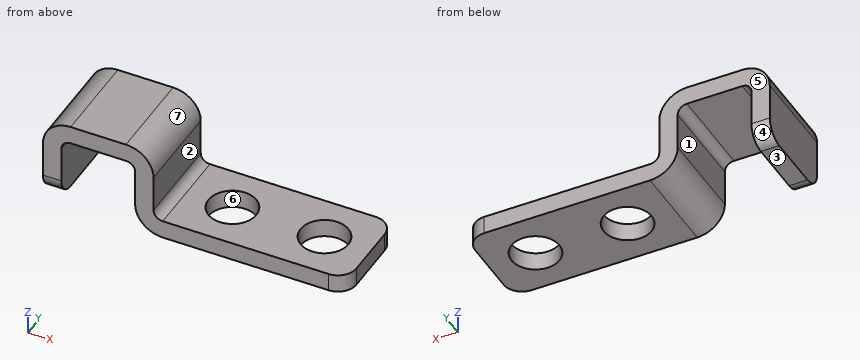
from build123d import *

# Parameters (mm, degrees)
F1_W = 10
F1_H = 2
F3_R = 2
F4_R = 2
F6_D = 5.2


with BuildPart() as f2:
    # F2: sweep along a path in F0
    with BuildLine(Plane.XZ) as f2_path:
        Line((0, 0), (-20, 0))
        ThreePointArc((-20, 0), (-21.4142135624, 0.5857864376), (-22, 2))
        Line((-22, 2), (-22, 6))
        ThreePointArc((-22, 6), (-22.5857864376, 7.4142135624), (-24, 8))
        Line((-24, 8), (-30, 8))
        ThreePointArc((-30, 8), (-31.4142135624, 7.4142135624), (-32, 6))
        Line((-32, 6), (-32, 0))
    # F1 (on Right) → F2 (sweep)
    with BuildSketch(Plane.YZ):
        with Locations((5, 0)):
            Rectangle(F1_W, F1_H)
    sweep(path=f2_path.line)

    # F3
    f3_edges = [f2.edges().sort_by_distance(p)[0] for p in [
        (-32, 0, 0),
        (-32, 10, 0),
    ]]
    fillet(f3_edges, radius=F3_R)

    # F4
    f4_edges = [f2.edges().sort_by_distance(p)[0] for p in [
        (0, 0, 0),
        (0, 10, 0),
    ]]
    fillet(f4_edges, radius=F4_R)

    # F6 (through all)
    with Locations(Plane.XY.offset(1)):
        with Locations((-15, 5), (-5, 5)):
            Hole(F6_D / 2)


solid = f2.part
The listing builds one solid part. Answer for the finished solid, in the listing's coordinates (mm). Face numbers are marked on the shaded views. A direction names the side the tool comes from. Coordinates: 2 decimals unless noted, no trailing zeros. Loops run counter-clockwise (first coordinate to the right, second up) from the corner with the lowest first, then second, coordinate; pieces in that order, holes last.
1) Determine the mould class of the marked faces 5, 6 and 7 for opening direction Y: pulls with the +Y half, pulls with the -Y half, needs draft (parallel to the pull), parting line crosses it, or undercut.
2) Find section A-A on x = -4. Write down the section's boundary in (y, z).
3) Find section B-B on y = 2.75. Write down the section's boundary in (x, z).
4) Flat-ended cylindrical pins translate along their axes: pin 1 Ø1.2 at (y, z) = (4.5, 3.5) entering from +X; pin 2 Ø2 at (x, y) = (-32.5, 6.5) entering from -Z; pin 3 Ø4 at (x, z) = (-26, 2.5) entering from -Y; pin 4 Ø3 at (x, y) = (-12, 5.5) entering from +Z. Find the tip coordinate at first contact, or state that the pin passes through.
5) Find section D-D on y = 6. Write down the section's boundary in (x, z).
6) Find section C-C on z = 6.5. Write down the section's boundary in (x, y).
7) Find the intervals of material crossed by L1, parallel to X at y = 0.5, z = 4; L2, parallel to Y at x = -5, z = 0.25; L3, parallel to Z at x = -29, y = 7, in increasing order.
8) A tool of negligible diameter and unlimited length cuts with its end or side. For the marked faces 1, 2, 3 and 4, from which of +Z, -Z, +X, -X, +Y, -Y can it reach the whole face along a straight path? Write none if from no direction.
Values:
1. face 5: pulls with the +Y half
1. face 6: undercut
1. face 7: needs draft
2. outline: (0, -1) - (2.6, -1) - (2.6, 1) - (0, 1) - close; (7.4, -1) - (10, -1) - (10, 1) - (7.4, 1) - close
3. outline: (-33, 0) - (-31, 0) - (-31, 6) arc R1 cw to (-30, 7) - (-24, 7) arc R1 cw to (-23, 6) - (-23, 2) arc R3 ccw to (-20, -1) - (-16.3, -1) - (-16.3, 1) - (-20, 1) arc R1 cw to (-21, 2) - (-21, 6) arc R3 ccw to (-24, 9) - (-30, 9) arc R3 ccw to (-33, 6) - close; (-13.7, -1) - (-6.3, -1) - (-6.3, 1) - (-13.7, 1) - close; (-3.7, -1) - (0, -1) - (0, 1) - (-3.7, 1) - close
4. pin 1: stops at x = -21
4. pin 2: stops at z = 0
4. pin 3: passes through
4. pin 4: stops at z = 1
5. outline: (-33, 0) - (-31, 0) - (-31, 6) arc R1 cw to (-30, 7) - (-24, 7) arc R1 cw to (-23, 6) - (-23, 2) arc R3 ccw to (-20, -1) - (-17.4, -1) - (-17.4, 1) - (-20, 1) arc R1 cw to (-21, 2) - (-21, 6) arc R3 ccw to (-24, 9) - (-30, 9) arc R3 ccw to (-33, 6) - close; (-12.6, -1) - (-7.4, -1) - (-7.4, 1) - (-12.6, 1) - close; (-2.6, -1) - (0, -1) - (0, 1) - (-2.6, 1) - close
6. outline: (-32.96, 0) - (-30.87, 0) - (-30.87, 10) - (-32.96, 10) - close; (-23.13, 0) - (-21.04, 0) - (-21.04, 10) - (-23.13, 10) - close
7. L1: x = -33 to -31, -23 to -21
7. L2: y = 0 to 2.4, 7.6 to 10
7. L3: z = 7 to 9
8. face 1: -Z, +Y, -Y
8. face 2: +Z, +X, +Y, -Y
8. face 3: -Z, -X, +Y, -Y
8. face 4: -Z, -X, +Y
